from build123d import *

# Parameters (mm, degrees)
EXTRUDE_1_DEPTH     = 2
SKETCH_2_R          = 2.5
CUT_EXTRUDE_3_DEPTH = 3
SKETCH_3_R          = 1.5
EXTRUDE_2_DEPTH     = 4
SKETCH_4_R          = 0.75
EXTRUDE_3_DEPTH     = 5
SKETCH_5_W          = 40
SKETCH_5_H          = 4.5
EXTRUDE_4_DEPTH     = 2
SKETCH_6_R          = 0.5
CUT_EXTRUDE_4_DEPTH = 1
SKETCH_7_R          = 2
CUT_EXTRUDE_5_DEPTH = 3


with BuildPart() as part:
    # 草图1 → 凸台-拉伸1 (new body)
    with BuildSketch(Plane.XY):
        Polygon((-21.685600323, 10.142561447), (18.314399677, 10.142561447), (28.314399677, -9.857438553), (28.314399677, -18.857438553), (18.314399677, -18.857438553), (18.314399677, -9.857438553), (-21.685600323, -9.857438553), (-21.685600323, -18.857438553), (-31.685600323, -18.857438553), (-31.685600323, -9.857438553), align=None)
    extrude(amount=EXTRUDE_1_DEPTH)

    # 草图2 → 切除-拉伸3 (cut, through all)
    with BuildSketch(Plane.XY):
        with Locations((-26.685600323, -14.857438553)):
            Circle(SKETCH_2_R)
        with Locations((23.314399677, -14.857438553)):
            Circle(SKETCH_2_R)
    extrude(amount=CUT_EXTRUDE_3_DEPTH, mode=Mode.SUBTRACT)

    # 草图3 → 凸台-拉伸2 (add)
    with BuildSketch(Plane(origin=(0, 0, 0), x_dir=(-1, 0, 0), z_dir=(0, 0, -1))):
        with Locations((-16.314399677, 5.142561447)):
            Circle(SKETCH_3_R)
        with Locations((19.685600323, 5.142561447)):
            Circle(SKETCH_3_R)
    extrude(amount=EXTRUDE_2_DEPTH)

    # 草图4 → 凸台-拉伸3 (add)
    with BuildSketch(Plane(origin=(0, 0, -4), x_dir=(-1, 0, 0), z_dir=(0, 0, -1))):
        with Locations((-16.314399677, 5.142561447)):
            Circle(SKETCH_4_R)
        with Locations((19.685600323, 5.142561447)):
            Circle(SKETCH_4_R)
    extrude(amount=EXTRUDE_3_DEPTH)

    # 草图5 → 凸台-拉伸4 (add)
    with BuildSketch(Plane.XY):
        with Locations((-1.685600323, -12.107438553)):
            Rectangle(SKETCH_5_W, SKETCH_5_H)
    extrude(amount=EXTRUDE_4_DEPTH)

    # 草图6 → 切除-拉伸4 (cut)
    with BuildSketch(Plane.XY.offset(2)):
        with Locations((-23.685600323, -7.357438553)):
            Circle(SKETCH_6_R)
        with Locations((20.314399677, -7.357438553)):
            Circle(SKETCH_6_R)
        with Locations((-19.685600323, -2.357438553)):
            Circle(SKETCH_6_R)
        with Locations((16.314399677, -2.357438553)):
            Circle(SKETCH_6_R)
    extrude(amount=-CUT_EXTRUDE_4_DEPTH, mode=Mode.SUBTRACT)

    # 草图7 → 切除-拉伸5 (cut, through all)
    with BuildSketch(Plane(origin=(0, 0, 0), x_dir=(-1, 0, 0), z_dir=(0, 0, -1))):
        with Locations((1.818081587, -1.181083472)):
            Circle(SKETCH_7_R)
    extrude(amount=-CUT_EXTRUDE_5_DEPTH, mode=Mode.SUBTRACT)


solid = part.part
Source: CAD feature listing. Evaluate the final solid. Frame: model axes, mm. A direction names the side the tool comes from. Round coordinates to 2 decimals unless told otherwise and drop trailing zeros. Order: outer loops, then holes, each group sorted by start corner. A loop starts at its lowest first (then second) coordinate and runs counter-clockwise, first axis right, second up. Notation, with made-up numbers: (-9.5, 63) - (41.5, 63) arc R17 ccw to (41.5, 93) - close; hole circle Ø7 at (41, 25). An arc over 180 degrees is marked (long way). Use a Markdown table: item, result. Add a question column.
1. Section query D-D (x = -26). Return the cut outline in (y, z), then the cut area to 3 significant figures.
2. Section query C-C (z = -2.25). Return the cut outline in (x, y).
3. Mould query, pull axis X, two halves, no side actions, for faces 1 (the flat face through (23.244, 0.283, 0.986)), 2 (the flat face through (-2, -4, 2)), 3 (the cylindrical face through (-19.09, 4.69, -6.46)), 4 (the cylindrical face through (24.66, -12.75, 0.99)). Classes: +X half, -X half, draft (parallel to the pull), parting line (faces both ways), or undercut.
4. First-contact query: pin 1 (1 mm diameter, centred on x = -5.5, y = 4, fed in from -Z); pin 2 (3 mm diameter, centred on x = -26.69, y = -14.86, fed in from -Z); pin 3 (1.1 mm diameter, centred on x = -23.5, y = -7.5, fed in from +Z); pin 4 (3 mm diameter, centred on y = 3.5, z = -7, fed in from +X). Flat tips, straight axial feed; report the tip coordinate or a pass-through.
5. Section query B-B (y = -15.75). Return the cut outline in (x, z), then the cut area to 3 significant figures.
6. Section query A-A (x = -1). Return the cut outline in (y, z).
7. Set-up query: faces 5 (the flat face through (-2, -14.357, 1)), 6 (the cylindrical face through (-18.187, 5.209, -1.972)), 7 (the flat face through (-31.686, -14, 1)). Return all of +Z, -Z, +X, -X, +Y, -Y with unobstructed straight access to the full face (end or side cutting, diameter ignored); none if empty.
8. Line query: probe 1 along X at (y, z) = (-14.25, 0.5); probe 2 along X at (y, z) = (5, -1.5); probe 3 along Z at (x, y) = (-22, -1). Output: solid intervals per line, ascending.
Derived:
| question | item | result |
|---|---|---|
| 1 | outline | (-18.86, 0) - (-17.26, 0) - (-17.26, 2) - (-18.86, 2) - close; (-12.45, 0) - (1.51, 0) - (1.51, 2) - (-12.45, 2) - close |
| 1 | area | 31.1 mm2 |
| 2 | outline | circle Ø3 at (-19.69, 5.14); circle Ø3 at (16.31, 5.14) |
| 3 | face 1 | +X half |
| 3 | face 2 | draft |
| 3 | face 3 | undercut |
| 3 | face 4 | undercut |
| 4 | pin 1 | z = 0 |
| 4 | pin 2 | through |
| 4 | pin 3 | z = 2 |
| 4 | pin 4 | x = 17.05 |
| 5 | outline | (-31.69, 0) - (-29.02, 0) - (-29.02, 2) - (-31.69, 2) - close; (-24.35, 0) - (-21.69, 0) - (-21.69, 2) - (-24.35, 2) - close; (18.31, 0) - (20.98, 0) - (20.98, 2) - (18.31, 2) - close; (25.65, 0) - (28.31, 0) - (28.31, 2) - (25.65, 2) - close |
| 5 | area | 21.3 mm2 |
| 6 | outline | (-14.36, 0) - (-3.01, 0) - (-3.01, 2) - (-14.36, 2) - close; (0.64, 0) - (10.14, 0) - (10.14, 2) - (0.64, 2) - close |
| 7 | face 5 | +Z, -Z, -Y |
| 7 | face 6 | -Z |
| 7 | face 7 | +Z, -Z, -X, +Y, -Y |
| 8 | probe 1 | -31.69 to -29.11, -24.26 to 20.89, 25.74 to 28.31 |
| 8 | probe 2 | -21.18 to -18.19, 14.82 to 17.81 |
| 8 | probe 3 | 0 to 2 |
